```python
from build123d import *

# Parameters (mm, degrees)
SKETCH_1_W = 100
SKETCH_1_H = 3
SKETCH_2_W = 62
SKETCH_2_H = 3


with BuildPart() as part:
    # 草图1 → 旋转1 (revolve)
    with BuildSketch(Plane.XY, mode=Mode.PRIVATE) as revolve_1_sk:
        with Locations((0, 1.5)):
            Rectangle(SKETCH_1_W, SKETCH_1_H)
    revolve(revolve_1_sk.sketch.rotate(Axis((-50, 0, 0), (1, 0, 0)), 90), axis=Axis((-50, 0, 0), (1, 0, 0)))

    # 草图2 → 旋转3 (revolve)
    with BuildSketch(Plane(origin=(0, 0, 0), x_dir=(0, 0, -1), z_dir=(1, 0, 0)), mode=Mode.PRIVATE) as revolve_3_sk:
        with Locations((0, 1.5)):
            Rectangle(SKETCH_2_W, SKETCH_2_H)
    revolve(revolve_3_sk.sketch.rotate(Axis((0, 0, 31), (0, 0, -1)), 90), axis=Axis((0, 0, 31), (0, 0, -1)))


solid = part.part
```
Model file for the job. Use its own axes, mm. A direction names the side the tool comes from. Give positions to 0.01 mm unless a question says otherwise; leave off trailing zeros. Write each loop counter-clockwise with the first axis right and the second up, starting at its lowest first coordinate (ties: lowest second). Pieces come first, ordered by that corner, then holes. Notation, with made-up numbers: (-6.5, -27) -> (0.5, -27) arc R4 ccw to (0.5, -23) -> close; hole circle Ø2 at (33.5, 25.25). An arc over 180 degrees is marked (long way). Use CSV: the item, a comma, the result in double quotes. Start each with the question number.
1) Drill centre lines: L1, parallel to Z at x = -19.5, y = 0.5; L2, parallel to X at y = 1.8, z = 28; L3, parallel to Z at x = -27, y = -0.8. Where is each one in solid material? Low to high.
2) Cut at B-B on x = -38. List the corners of the cut face in (y, z).
3) Tool access for faces 1 (the cylindrical face through (-25, 0, -3)), 2 (the cylindrical face through (25.35, -0.9, 2.86)), 3 (the cylindrical face through (1.384, 2.662, 15.283)), 4 (the cylindrical face through (2.86, -0.9, -15.72)): list every direction of +Z, -Z, +X, -X, +Y, -Y with a clear straight run to the whole face (end or side of a thin tool).
4) Cut at A-A on y = 0. List the corners of the cut face in (x, z), plus the area to 3 significant figures.
Final values:
1,L1,"z = -2.96 to 2.96"
1,L2,"x = -2.4 to 2.4"
1,L3,"z = -2.89 to 2.89"
2,outline,"circle Ø6 at (0, 0)"
3,face 1,"-X"
3,face 2,"+X"
3,face 3,"+Z"
3,face 4,"-Z"
4,outline,"(-50, -3) -> (-3, -3) -> (-3, -31) -> (3, -31) -> (3, -3) -> (50, -3) -> (50, 3) -> (3, 3) -> (3, 31) -> (-3, 31) -> (-3, 3) -> (-50, 3) -> close"
4,area,"936 mm2"
